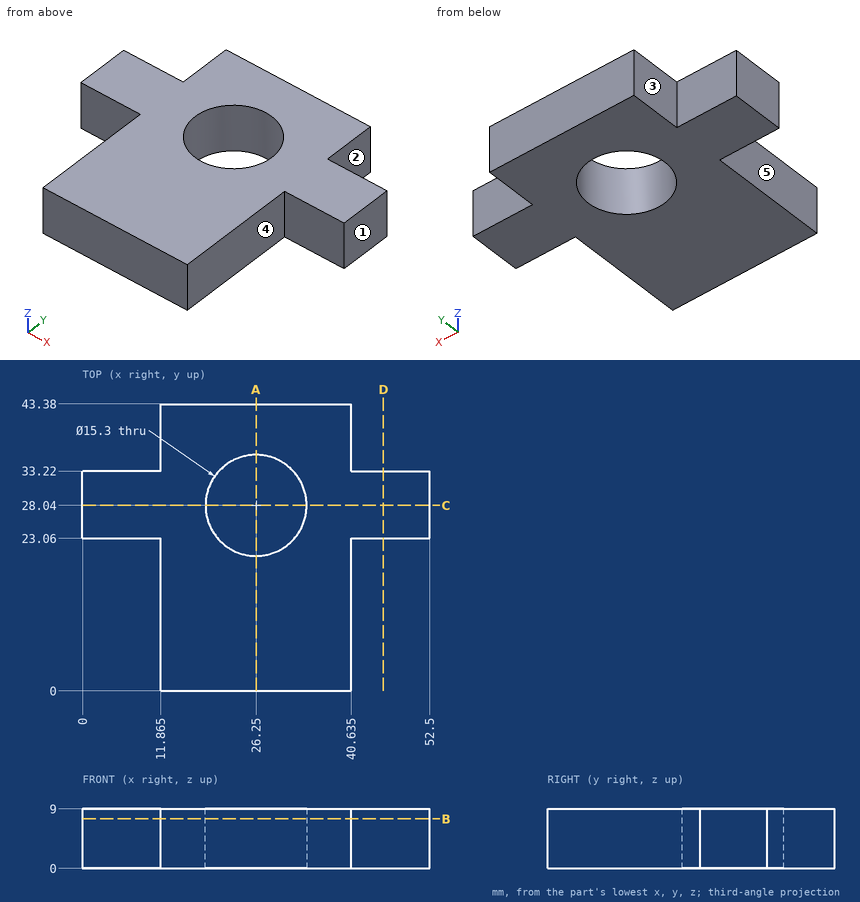
The drawing under review shows one solid part. Ordinate dimensions are in mm from its lowest x, y, z. A direction names the side the tool comes from. Give positions to 0.01 mm unless a question says otherwise; leave off trailing zeros. Write each loop counter-clockwise with the first axis right and the second up, starting at its lowest first coordinate (ties: lowest second). Pieces come first, ordered by that corner, then holes. Notation, with made-up numbers: (31, 47.5) -> (72, 47.5) arc R32 cw to (72, 85.5) -> close; hole circle Ø1 at (-24.75, -30). An arc over 180 degrees is marked (long way). Answer in a Markdown table with one row per item.
(1) To check wall thickness, follow probe 1 along Y at (x, z) = (26.25, 3.75); probe 2 along X at (y, z) = (38, 2.5) (3 decimals); probe 3 along Y at (x, z) = (45, 2). State the ranges of each line that lie inside material, in increasing order.
Results:
| item | result |
|---|---|
| probe 1 | 0 to 20.39, 35.69 to 43.38 |
| probe 2 | 11.865 to 40.635 |
| probe 3 | 23.06 to 33.22 |
(2) Consider section B-B (z = 7.5). State the section outline as (x, y) points (3 decimals).
Results:
| item | result |
|---|---|
| outline | (0, 23.06) -> (11.865, 23.06) -> (11.865, 0) -> (40.635, 0) -> (40.635, 23.06) -> (52.5, 23.06) -> (52.5, 33.22) -> (40.635, 33.22) -> (40.635, 43.38) -> (11.865, 43.38) -> (11.865, 33.22) -> (0, 33.22) -> close; hole circle Ø15.3 at (26.25, 28.04) |
(3) Consider section A-A (x = 26.25). State the section outline as (y, z) points, then the cut area to 3 significant figures.
Results:
| item | result |
|---|---|
| outline | (0, 0) -> (20.39, 0) -> (20.39, 9) -> (0, 9) -> close; (35.69, 0) -> (43.38, 0) -> (43.38, 9) -> (35.69, 9) -> close |
| area | 253 mm2 |
(4) Consider section C-C (y = 28.04). State the section outline as (x, z) points, then the cut area to 3 significant figures.
Results:
| item | result |
|---|---|
| outline | (0, 0) -> (18.6, 0) -> (18.6, 9) -> (0, 9) -> close; (33.9, 0) -> (52.5, 0) -> (52.5, 9) -> (33.9, 9) -> close |
| area | 335 mm2 |
(5) For the marked faces 1, 2, 3, 4 and 5, list the 3-axis set-ups (+Z, -Z, +X, -X, +Y, -Y) from which the entire face can be reached by the end or side of a thin tool; tool diameter is ignored.
Results:
| item | result |
|---|---|
| face 1 | +Z, -Z, +X, +Y, -Y |
| face 2 | +Z, -Z, +X, +Y |
| face 3 | +Z, -Z, -X, +Y |
| face 4 | +Z, -Z, +X, -Y |
| face 5 | +Z, -Z, -X, -Y |
(6) Consider section D-D (x = 45.5). State the section outline as (y, z) points.
Results:
| item | result |
|---|---|
| outline | (23.06, 0) -> (33.22, 0) -> (33.22, 9) -> (23.06, 9) -> close |
(7) Clearance check with flat-ended pins moving along their axes: pin 1 (1 mm diameter, centred on y = 11.5, z = 3.5, fed in from +X) (3 decimals); pin 2 (4 mm diameter, centred on y = 37.5, z = 2.5, fed in from -X) (3 decimals); pin 3 (4.5 mm diameter, centred on x = 7.5, z = 5, fed in from -Y); pin 4 (3 mm diameter, centred on y = 27, z = 2.5, fed in from -X). State where each tip first meets the part, or that it passes through.
Results:
| item | result |
|---|---|
| pin 1 | x = 40.635 |
| pin 2 | x = 11.865 |
| pin 3 | y = 23.06 |
| pin 4 | x = 0 |
